Source: CAD feature listing. Evaluate the final solid. Frame: model axes, mm. A direction names the side the tool comes from. Round coordinates to 2 decimals unless told otherwise and drop trailing zeros. Order: outer loops, then holes, each group sorted by start corner. A loop starts at its lowest first (then second) coordinate and runs counter-clockwise, first axis right, second up. Notation, with made-up numbers: M 5.5,0 L 31.5,0 A19 cw 31.5,37 Z; hole C -26.5,1 d10. An arc over 180 degrees is marked long. Use one line per item in the form item = value. Start each with the question number.
Q1. Section C-C (z = 0). Return the cut outline in (x, y).
Q2. Section D-D (y = 46). Return the cut outline in (x, z).
Q3. Section B-B (y = 60). Return the cut outline in (x, z).
Q4. Section A-A (x = 0). Return the cut outline in (y, z).
Q5. Material intervals for probe 1 along X at (y, z) = (20.5, 0); probe 2 along Y at (x, z) = (2.75, 2.25); probe 3 along X at (y, z) = (51, 4.5), sorted ascending.
Q6. Reachability of faces 1 (the cylindrical face through (-4.88, 24.65, -1.08)), 2 (the flat face through (-10, 60, 0)), 3 (the cylindrical face through (15, 64, -3)) from +Z, -Z, +X, -X, +Y, -Y: full face, straight path, thin tool, end or side. Return the list, or none.
Q7. Pull-direction query (X, two-part tool) for faces 4 (the flat face through (20, 60, 0)), 5 (the flat face through (0, 50, 0)), 6 (the flat face through (0, 60, 10)); classes: pulls with the +X half, pulls with the -X half, needs draft (parallel to the pull), parting line crosses it, or undercut.
Q8. Contact query for flat-ended pins moving along their axis: pin 1 (6 mm diameter, centred on x = 2.5, y = 17.5, fed in from +Z); pin 2 (4 mm diameter, centred on y = 42.5, z = -0.5, fed in from -X); pin 3 (8 mm diameter, centred on x = -1.5, z = 1, fed in from -Y); pin 4 (3 mm diameter, centred on x = 10.5, z = -4.5, fed in from -Y). Output: stop coordinate, or through.
from build123d import *

# Parameters (mm, degrees)
SKETCH1_R           = 7.5
SKETCH1_R_2         = 5
BOSS_EXTRUDE1_DEPTH = 50
SKETCH3_W           = 20
SKETCH3_H           = 20
SKETCH3_R           = 7.5
SKETCH3_R_2         = 5
BOSS_EXTRUDE2_DEPTH = 20
SKETCH4_R           = 5
BOSS_EXTRUDE3_DEPTH = 10


with BuildPart() as part:
    # Sketch1 → Boss-Extrude1 (new body)
    with BuildSketch(Plane(origin=(0, 0, 0), x_dir=(1, 0, 0), z_dir=(0, 1, 0))):
        with Locations(Location((0, 0, 0), (0, 0, 270))):
            Circle(SKETCH1_R)
        with Locations(Location((0, 0, 0), (0, 0, 270))):
            Circle(SKETCH1_R_2, mode=Mode.SUBTRACT)
    extrude(amount=BOSS_EXTRUDE1_DEPTH)

    # Sketch3 → Boss-Extrude2 (add)
    # profile 1 of 3: a face of its own
    with BuildSketch(Plane(origin=(0, 50, 0), x_dir=(1, 0, 0), z_dir=(0, 1, 0))):
        Rectangle(SKETCH3_W, SKETCH3_H)
        with Locations(Location((0, 0, 0), (0, 0, 270))):
            Circle(SKETCH3_R, mode=Mode.SUBTRACT)
    # profile 2 of 3: a face of its own
    with BuildSketch(Plane(origin=(0, 50, 0), x_dir=(1, 0, 0), z_dir=(0, 1, 0))):
        with Locations(Location((0, 0, 0), (0, 0, 270))):
            Circle(SKETCH3_R)
        with Locations(Location((0, 0, 0), (0, 0, 270))):
            Circle(SKETCH3_R_2, mode=Mode.SUBTRACT)
    # profile 3 of 3: a face of its own
    with BuildSketch(Plane(origin=(0, 50, 0), x_dir=(1, 0, 0), z_dir=(0, 1, 0))):
        with Locations(Location((0, 0, 0), (0, 0, 270))):
            Circle(SKETCH3_R_2)
    extrude(amount=BOSS_EXTRUDE2_DEPTH)

    # Sketch4 → Boss-Extrude3 (add)
    with BuildSketch(Plane(origin=(10, 0, 0), x_dir=(0, 0, -1), z_dir=(1, 0, 0))):
        with Locations((0, 60)):
            Circle(SKETCH4_R)
    extrude(amount=BOSS_EXTRUDE3_DEPTH)


solid = part.part
Results list:
q1.outline = M -10,50 L -7.5,50 L -7.5,0 L -5,0 L -5,50 L 5,50 L 5,0 L 7.5,0 L 7.5,50 L 10,50 L 10,55 L 20,55 L 20,65 L 10,65 L 10,70 L -10,70 Z
q2.outline = C 0,0 d15; hole C 0,0 d10
q3.outline = M -10,-10 L 10,-10 L 10,-5 L 20,-5 L 20,5 L 10,5 L 10,10 L -10,10 Z
q4.outline = M 0,-7.5 L 50,-7.5 L 50,-10 L 70,-10 L 70,10 L 50,10 L 50,7.5 L 0,7.5 L 0,5 L 50,5 L 50,-5 L 0,-5 Z
q5.probe_1 = -7.5 to -5, 5 to 7.5
q5.probe_2 = 50 to 70
q5.probe_3 = -10 to 10
q6.face_1 = -Y
q6.face_2 = +Z, -Z, -X, +Y, -Y
q6.face_3 = +X
q7.face_4 = pulls with the +X half
q7.face_5 = undercut
q7.face_6 = needs draft
q8.pin_1 = 7.5
q8.pin_2 = -7.5
q8.pin_3 = 0
q8.pin_4 = 50
